```python
from build123d import *

# Parameters (mm, degrees)
PAD_DEPTH              = 66
SKETCH001_W            = 32.5
SKETCH001_H            = 40.15
PAD001_DEPTH           = 1.5
PAD002_DEPTH           = 1.2
PAD003_DEPTH           = 16
SKETCH011_W            = 16.471436
SKETCH011_H            = 30.415474
POCKET_DEPTH           = 5
POCKET001_DEPTH        = 13
POCKET002_DEPTH        = 5
LINEARPATTERN_COUNT    = 2
LINEARPATTERN_PITCH    = 31
POCKET003_DEPTH        = 32.501
LINEARPATTERN001_COUNT = 2
LINEARPATTERN001_PITCH = 29
SKETCH017_W            = 17
SKETCH017_H            = 34.922093
POCKET004_DEPTH        = 5
FILLET_R               = 3
FILLET001_R            = 1
FILLET002_R            = 2
FILLET003_R            = 2
FILLET004_R            = 1
FILLET005_R            = 1


with BuildPart() as part:
    # Sketch → Pad (new body)
    with BuildSketch(Plane.XY):
        Polygon((14.75, 37.75), (14.75, 0), (-14.75, 0), (-14.75, 37.75), (-12.25, 37.75), (-12.25, 38.95), (-16.25, 38.95), (-16.25, -1.2), (16.25, -1.2), (16.25, 38.95), (12.25, 38.95), (12.25, 37.75), align=None)
    extrude(amount=PAD_DEPTH)

    # Sketch001 (on Face13 of Pad) → Pad001 (join)
    with BuildSketch(Plane(origin=(0, 0, 0), x_dir=(1, 0, 0), z_dir=(0, 0, -1))):
        with Locations((0, -18.875)):
            Rectangle(SKETCH001_W, SKETCH001_H)
    extrude(amount=PAD001_DEPTH)

    # Sketch002 (on Face13 of Pad001) → Pad002 (join)
    with BuildSketch(Plane.XZ.offset(1.2)):
        Polygon((-16.25, 66), (-4, 94), (4, 94), (16.25, 66), align=None)
    extrude(amount=-PAD002_DEPTH)

    # Sketch007 (on Face8 of Pad002) → Pad003 (join)
    with BuildSketch(Plane(origin=(0, 0, 0), x_dir=(-1, 0, 0), z_dir=(0, 1, 0))):
        Polygon((-16.25, 66), (-15, 66), (-3.5, 88), (3.5, 88), (15, 66), (16.25, 66), (4, 94), (-4, 94), align=None)
    extrude(amount=PAD003_DEPTH)

    # Sketch011 (on Face24 of Pad003) → Pocket (cut)
    with BuildSketch(Plane(origin=(37.87541, 0, 16.570492), x_dir=(0, 1, 0), z_dir=(0.916157, 0, 0.400819))):
        with Locations((0, -31.207737)):
            Rectangle(SKETCH011_W, SKETCH011_H)
    extrude(amount=-POCKET_DEPTH, mode=Mode.SUBTRACT)

    # Sketch016 (on Face27 of Pocket) → Pocket001 (cut)
    with BuildSketch(Plane.XY.offset(94)):
        with BuildLine():
            ThreePointArc((3, 13.5), (0, 16.5), (-3, 13.5))
            Line((-3, 13.5), (-3, 11))
            ThreePointArc((-3, 11), (0, 8), (3, 11))
            Line((3, 13.5), (3, 11))
        make_face()
    extrude(amount=-POCKET001_DEPTH, mode=Mode.SUBTRACT)

    # Sketch014 (on Face23 of Pocket001) → Pocket002 (cut)
    with BuildSketch(Plane.XZ.offset(1.2)):
        Polygon((0, 22.534029), (-8, 13), (-8, 5), (8, 5), (8, 13), align=None)
    pocket002 = extrude(amount=-POCKET002_DEPTH, mode=Mode.SUBTRACT)

    # LinearPattern: Pocket002 ×2
    with Locations(*[(0, 0, i * LINEARPATTERN_PITCH) for i in range(1, LINEARPATTERN_COUNT)]):
        add(pocket002, mode=Mode.SUBTRACT)

    # Sketch015 (on Face23 of LinearPattern) → Pocket003 (cut, through all)
    with BuildSketch(Plane.YZ.offset(16.25)):
        Polygon((18.770192, 29.113804), (8.770192, 18.200719), (8.770192, 7.200719), (28.770192, 7.200719), (28.770192, 18.200719), align=None)
    pocket003 = extrude(amount=-POCKET003_DEPTH, mode=Mode.SUBTRACT)

    # LinearPattern001: Pocket003 ×2
    with Locations(*[(0, 0, i * LINEARPATTERN001_PITCH) for i in range(1, LINEARPATTERN001_COUNT)]):
        add(pocket003, mode=Mode.SUBTRACT)

    # Sketch017 (on Face50 of LinearPattern001) → Pocket004 (cut)
    with BuildSketch(Plane(origin=(0, 0, -1.5), x_dir=(1, 0, 0), z_dir=(0, 0, -1))):
        with Locations((0, -34.411046)):
            Rectangle(SKETCH017_W, SKETCH017_H)
    extrude(amount=-POCKET004_DEPTH, mode=Mode.SUBTRACT)

    # Fillet
    fillet_edges = [part.edges().sort_by_distance(p)[0] for p in [
        (-8.5, 38.95, -0.75),
        (8.5, 38.95, -0.75),
    ]]
    fillet(fillet_edges, radius=FILLET_R)

    # Fillet001
    fillet001_edges = [part.edges().sort_by_distance(p)[0] for p in [
        (-8.5, 16.95, -0.75),
    ]]
    fillet(fillet001_edges, radius=FILLET001_R)

    # Fillet002
    fillet002_edges = [part.edges().sort_by_distance(p)[0] for p in [
        (-16.25, 38.95, 33),
        (16.25, 38.95, 33),
    ]]
    fillet(fillet002_edges, radius=FILLET002_R)

    # Fillet003
    fillet003_edges = [part.edges().sort_by_distance(p)[0] for p in [
        (-14.75, 37.75, 33),
        (14.75, 37.75, 33),
    ]]
    fillet(fillet003_edges, radius=FILLET003_R)

    # Fillet004
    fillet004_edges = [part.edges().sort_by_distance(p)[0] for p in [
        (4, 8, 94),
    ]]
    fillet(fillet004_edges, radius=FILLET004_R)

    # Fillet005
    fillet005_edges = [part.edges().sort_by_distance(p)[0] for p in [
        (-4, 8, 94),
    ]]
    fillet(fillet005_edges, radius=FILLET005_R)


solid = part.part
```
Check sheet for the modelled part. Datum: model origin and axes. Units: mm. A direction names the side the tool comes from. Round coordinates to 2 decimals unless told otherwise and drop trailing zeros. Order: outer loops, then holes, each group sorted by start corner. A loop starts at its lowest first (then second) coordinate and runs counter-clockwise, first axis right, second up. Notation, with made-up numbers: (53.25, -12) - (64.25, -12) arc R8 ccw to (64.25, -6) - close; hole circle Ø3 at (-31, 3.5). An arc over 180 degrees is marked (long way). Answer as CSV lines item,"result". Start each with the question number.
1) Section check C-C (z = 35). Record the cut outline in (x, y), then the cut area to 3 significant figures.
2) Tool access check on faces 5 (the face through (4.056, -0.608, 48.7)), 6 (the face through (3, 12, 91)), 7 (the face through (9.33, 7.89, 76.85)), 8 (the face through (-15.49, 13.84, 52.734)), 9 (the face through (0, 15, 0)). Record the directions out of +Z, -Z, +X, -X, +Y, -Y that give a thin tool (end or side, any length) a straight path to the whole face; none if there is none.
3) Scan lines: probe 1 along X at (y, z) = (25.5, 36); probe 2 along Y at (x, z) = (-8, 68); probe 3 along Z at (x, y) = (-12, 37). Record each from-to range of solid material in increasing order.
4) Draft check along Y on faces 1 (the face through (15.51, 13.84, 52.734)), 2 (the face through (-9.17, 7.89, 77.15)), 3 (the face through (13, 38.95, 33)), 4 (the face through (15.51, 23.84, 52.58)). Enter one of: +Y half, -Y half, draft (parallel to the pull), parting line (faces both ways), or undercut.
5) Section check A-A (z = 15). Record the cut outline in (x, y), then the cut area to 3 significant figures.
6) Section check B-B (x = -10.5). Record the cut outline in (y, z), then the cut area to 3 significant figures.
7) Depth check by flat-ended pin: pin 1 (1.3 mm diameter, centred on y = 38.5, z = 44, fed in from -X); pin 2 (6 mm diameter, centred on x = 8, y = 11, fed in from +Z); pin 3 (12 mm diameter, centred on x = 3.5, z = 80.5, fed in from +Y). Enter the tip coordinate at first touch or a pass-through.
Determined:
1,outline,"(-16.25, -1.2) - (16.25, -1.2) - (16.25, 36.95) arc R2 ccw to (14.25, 38.95) - (12.25, 38.95) - (12.25, 37.75) - (12.75, 37.75) arc R2 cw to (14.75, 35.75) - (14.75, 0) - (-14.75, 0) - (-14.75, 35.75) arc R2 cw to (-12.75, 37.75) - (-12.25, 37.75) - (-12.25, 38.95) - (-14.25, 38.95) arc R2 ccw to (-16.25, 36.95) - close"
1,area,"162 mm^2"
2,face 5,"+Y, -Y"
2,face 6,"+Z"
2,face 7,"+Y"
2,face 8,"+X, -X"
2,face 9,"none"
3,probe 1,"-16.25 to -14.75, 14.75 to 16.25"
3,probe 2,"-1.2 to 0"
3,probe 3,"-1.5 to 0"
4,face 1,"undercut"
4,face 2,"draft"
4,face 3,"+Y half"
4,face 4,"undercut"
5,outline,"(-16.25, -1.2) - (-6.32, -1.2) - (-6.32, 0) - (-14.75, 0) - (-14.75, 8.77) - (-16.25, 8.77) - close; (-16.25, 28.77) - (-14.75, 28.77) - (-14.75, 35.75) arc R2 cw to (-12.75, 37.75) - (-12.25, 37.75) - (-12.25, 38.95) - (-14.25, 38.95) arc R2 ccw to (-16.25, 36.95) - close; (6.32, -1.2) - (16.25, -1.2) - (16.25, 8.77) - (14.75, 8.77) - (14.75, 0) - (6.32, 0) - close; (12.25, 37.75) - (12.75, 37.75) arc R2 cw to (14.75, 35.75) - (14.75, 28.77) - (16.25, 28.77) - (16.25, 36.95) arc R2 ccw to (14.25, 38.95) - (12.25, 38.95) - close"
5,area,"86.7 mm^2"
6,outline,"(-1.2, -1.5) - (38.78, -1.5) - (38.78, 0) - (0, 0) - (0, 74.61) - (16, 74.61) - (16, 79.14) - (-1.2, 79.14) - close"
6,area,"227 mm^2"
7,pin 1,"x = -16.04"
7,pin 2,"z = 91.71"
7,pin 3,"y = 16"
